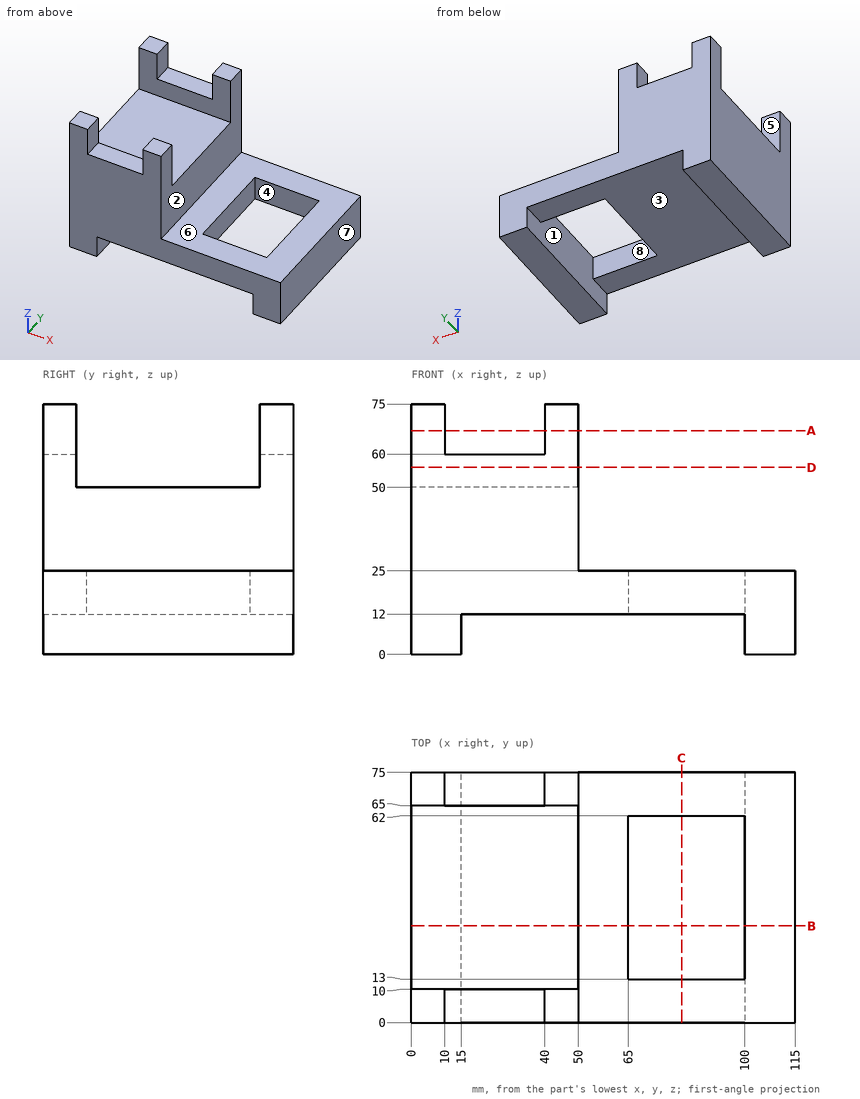
Geometry check sheet. Reference: drawing and pictorial views, mm from the part's lowest x, y, z. A direction names the side the tool comes from. Round coordinates to 2 decimals unless told otherwise and drop trailing zeros. Write each loop counter-clockwise with the first axis right and the second up, starting at its lowest first coordinate (ties: lowest second). Pieces come first, ordered by that corner, then holes.
1. Scan lines: L1, parallel to X at y = 67.5, z = 9; L2, parallel to X at y = 39, z = 17; L3, parallel to X at y = 46.5, z = 48. Record each from-to range of solid material in increasing order.
2. Gauge pin test, flat ends, axial feed: P1, Ø3, axis at x = 21.5, y = 5, coming from the +Z side; P2, Ø8, axis at y = 69, z = 65, coming from the +X side; P3, Ø15, axis at x = 35.5, y = 24.5, coming from the +Z side. Record the tip position at first contact, or that the pin passes through.
3. Section check C-C on x = 81. Enter the section's corners in (y, z), plus the area to 3 significant figures.
4. Draft check along X on the marked faces 6, 7 and 8. Enter one of: +X half, -X half, draft (parallel to the pull), parting line (faces both ways), or undercut.
5. Section check A-A on z = 67. Enter the section's corners in (x, y).
6. Section check D-D on z = 56. Enter the section's corners in (x, y).
7. Section check B-B on y = 29. Enter the section's corners in (x, z).
8. Access from +Z, -Z, +X, -X, +Y, -Y to the whole of each face (thin tool, end or side, straight path). Record for the marked faces 1, 2, 3, 4 and 5.
Answer:
1. L1: x = 0 to 15, 100 to 115
1. L2: x = 0 to 65, 100 to 115
1. L3: x = 0 to 50
2. P1: stops at z = 60
2. P2: stops at x = 50
2. P3: stops at z = 50
3. outline: (0, 12) - (13, 12) - (13, 25) - (0, 25) - close; (62, 12) - (75, 12) - (75, 25) - (62, 25) - close
3. area: 338 mm2
4. face 6: draft
4. face 7: +X half
4. face 8: undercut
5. outline: (0, 0) - (10, 0) - (10, 10) - (0, 10) - close; (0, 65) - (10, 65) - (10, 75) - (0, 75) - close; (40, 0) - (50, 0) - (50, 10) - (40, 10) - close; (40, 65) - (50, 65) - (50, 75) - (40, 75) - close
6. outline: (0, 0) - (50, 0) - (50, 10) - (0, 10) - close; (0, 65) - (50, 65) - (50, 75) - (0, 75) - close
7. outline: (0, 0) - (15, 0) - (15, 12) - (65, 12) - (65, 25) - (50, 25) - (50, 50) - (0, 50) - close; (100, 0) - (115, 0) - (115, 25) - (100, 25) - close
8. face 1: -Z
8. face 2: +Z, +X, +Y, -Y
8. face 3: -Z, +Y, -Y
8. face 4: +Z, -Z
8. face 5: +Z, +X, -X
